For this review, take the finished solid that the model builds, in its own axes (mm). Coordinates: 2 decimals unless noted, no trailing zeros. Loops run counter-clockwise (first coordinate to the right, second up) from the corner with the lowest first, then second, coordinate; pieces in that order, holes last. Notation, with made-up numbers: M 33.5,58 L 55.5,58 A26 ccw 55.5,88 Z; hole C -34.75,81 d5. An arc over 180 degrees is marked long. Put each result on its own line as item: value.
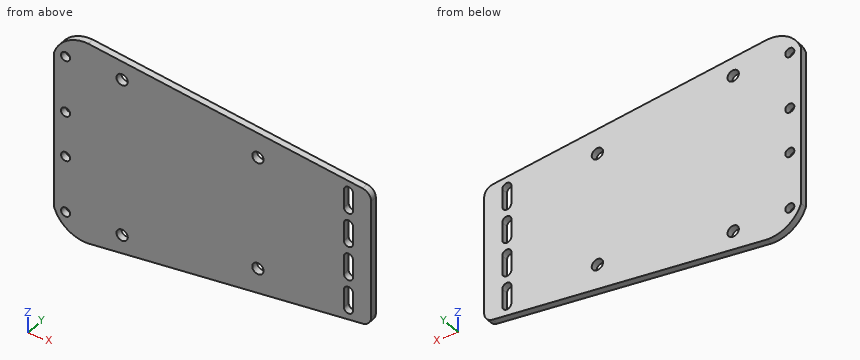
Autodesk Inventor part; units mm, degrees
ref_plane "YZ Plane" through (0, 0, 0) normal (1, 0, 0) x (0, 1, 0)
ref_plane "XZ Plane" through (0, 0, 0) normal (0, 1, 0) x (-1, 0, 0)
ref_plane "XY Plane" through (0, 0, 0) normal (0, 0, 1) x (1, 0, 0)
sketch "Boceto1" plane through (0, 0, 0) normal (0, 1, 0) x (-1, 0, 0)
  line L0 (125, 0) -> (125, 45)
  line L1 (140, 0) -> (140, 35)
  arc A0 (140, 35) -> (125, 45) centre (125.919, 30.1285) ccw
  line L2 (0, 0) -> (0, 26.2041)
  line L3 (10, 0) -> (10, 32.2222)
  line L4 (0, 0) -> (0, 7.5)
  line L5 (0, 7.5) -> (0, 22.5)
  arc A1 (8, 3.5) -> (12, 3.5) centre (10, 3.5) ccw
  line L6 (10, 7.5) -> (6.5727, 7.5)
  arc A2 (12, 11.5) -> (8, 11.5) centre (10, 11.5) ccw
  line L7 (10, 15) -> (5.5099, 15)
  line L8 (12, 11.5) -> (12, 3.5)
  line L9 (8, 3.5) -> (8, 11.5)
  arc A3 (12, 26.5) -> (8, 26.5) centre (10, 26.5) ccw
  arc A4 (8, 18.5) -> (12, 18.5) centre (10, 18.5) ccw
  line L10 (12, 18.5) -> (12, 26.5)
  line L11 (8, 26.5) -> (8, 18.5)
  circle A5 centre (135, 10) radius 2
  circle A6 centre (135, 35) radius 2
  circle A7 centre (110, 35) radius 2.5
  line L12 (125, 45) -> (3.7689, 30.4523)
  circle A8 centre (50, 25) radius 2.5
  arc A9 (3.7689, 30.4523) -> (0, 26.2041) centre (4.2786, 26.2041) ccw
  line L13 (0, 0) -> (10, 0)
  line L14 (125, 0) -> (125, -45)
  line L15 (140, 0) -> (140, -35)
  arc A10 (125, -45) -> (140, -35) centre (125.919, -30.1285) ccw
  line L16 (0, 0) -> (0, -26.2041)
  line L17 (10, 0) -> (10, -32.2222)
  line L18 (0, 0) -> (0, -7.5)
  line L19 (0, -7.5) -> (0, -22.5)
  arc A11 (12, -3.5) -> (8, -3.5) centre (10, -3.5) ccw
  line L20 (10, -7.5) -> (6.5727, -7.5)
  arc A12 (8, -11.5) -> (12, -11.5) centre (10, -11.5) ccw
  line L21 (10, -15) -> (5.5099, -15)
  line L22 (12, -11.5) -> (12, -3.5)
  line L23 (8, -3.5) -> (8, -11.5)
  arc A13 (12, -18.5) -> (8, -18.5) centre (10, -18.5) ccw
  line L24 (12, -18.5) -> (12, -26.5)
  line L25 (8, -26.5) -> (8, -18.5)
  arc A14 (8, -26.5) -> (12, -26.5) centre (10, -26.5) ccw
  circle A15 centre (135, -10) radius 2
  circle A16 centre (135, -35) radius 2
  circle A17 centre (110, -35) radius 2.5
  line L26 (125, -45) -> (3.7689, -30.4523)
  circle A18 centre (50, -25) radius 2.5
  arc A19 (0, -26.2041) -> (3.7689, -30.4523) centre (4.2786, -26.2041) ccw
  dimension "d15" = 45
  dimension "d18" = 15
  dimension "d19" = 35
  dimension "d24" = 140
  dimension "d27" = 10
  dimension "d28" = 7.5
  dimension "d29" = 15
  dimension "d32" = 4
  dimension "d33" = 4
  dimension "d34" = 5
  dimension "d35" = 5
  dimension "d36" = 35
  dimension "d37" = 10
  dimension "d38" = 4
  dimension "d39" = 4
  dimension "d40" = 35
  dimension "d41" = 30
  dimension "d42" = 5
  dimension "d43" = 25
  dimension "d44" = 50
  dimension "d45" = 96.843
  dimension "d51" = 5
extrude "Extrusión1" add sketch "Boceto1" along normal blind 3 contours L14 L26 L17 A14 L24 A13 A12 L22 A11 L3 A1 L8 A2 A4 L10 A3 L12 L0 | L0 A0 L1 L15 A10 L14 | L3 A3 L11 A4 A2 L9 A1 L13 L2 A9 L12 | L26 A19 L16 L13 L17 A11 L23 A12 A13 L25 A14
equation "\"d35\" = d34"
properties part number "SoporteMano"
(1) Add section B-B (x = -10). Write out the cut boundary in (y, z), plus the area to 3 significant figures.
Determined:
outline: M 0,-31.2 L 3,-31.2 L 3,-28.5 L 0,-28.5 Z; M 0,-16.5 L 3,-16.5 L 3,-13.5 L 0,-13.5 Z; M 0,-1.5 L 3,-1.5 L 3,1.5 L 0,1.5 Z; M 0,13.5 L 3,13.5 L 3,16.5 L 0,16.5 Z; M 0,28.5 L 3,28.5 L 3,31.2 L 0,31.2 Z
area: 43.2 mm^2
(2) Add section C-C (y = 0.6). State how many separate pieces and enclosed holes the cut face has, plus the area to 3 significant figures.
Determined:
separate pieces: 1
enclosed holes: 12
area: 10,300 mm^2
(3) Add section A-A (z = 5). Write out the cut boundary in (x, y).
Determined:
outline: M -140,0 L -12,0 L -12,3 L -140,3 Z; M -8,0 L 0,0 L 0,3 L -8,3 Z
(4) Add section D-D (x = -110). Write out the cut boundary in (y, z).
Determined:
outline: M 0,-43.2 L 3,-43.2 L 3,-37.5 L 0,-37.5 Z; M 0,-32.5 L 3,-32.5 L 3,32.5 L 0,32.5 Z; M 0,37.5 L 3,37.5 L 3,43.2 L 0,43.2 Z
(5) Wall thickness on line 1 along Z through (x, y) = (-135, 1.6); line 2 along Z through (x, y) = (-110, 0.7); line 3 along X through (y, z) = (0.85, -6): over which ranges is each line inside the solid? List them lowest first. Write a range as [from, to].
Determined:
line 1: z = [-41.94, -37], [-33, -12], [-8, 8], [12, 33], [37, 41.94]
line 2: z = [-43.2, -37.5], [-32.5, 32.5], [37.5, 43.2]
line 3: x = [-140, -12], [-8, 0]
(6) For pin 1 (4.5 mm diameter, centred on x = -110, z = 35, fed in from +Y), flat-tipped, find the tip position at first contact; note if it passes through.
Determined:
pin 1: passes through
